Autodesk Inventor part; units mm, degrees
ref_plane "YZ Plane" through (0, 0, 0) normal (1, 0, 0) x (0, 1, 0)
ref_plane "XZ Plane" through (0, 0, 0) normal (0, 1, 0) x (-1, 0, 0)
ref_plane "XY Plane" through (0, 0, 0) normal (0, 0, 1) x (1, 0, 0)
sketch "Sketch1" plane through (0, 0, 0) normal (1, 0, 0) x (0, 1, 0)
  circle A0 centre (0, 0) radius 4.953
  dimension "d0" = 9.906
extrude "Extrusion1" add sketch "Sketch1" along normal blind 0.635
sketch "Sketch2" plane through (0.635, 0, 0) normal (1, 0, 0) x (0, 0, -1)
  circle A0 centre (0, 0) radius 4.953
  circle A1 centre (0, 0) radius 3.4925
  dimension "d3" = 6.985
extrude "Extrusion2" cut sketch "Sketch2" against normal blind 0.381 contours A1
sketch "Sketch3" plane through (0.254, 0, 0) normal (1, 0, 0) x (0, 0, -1)
  circle A0 centre (0, 0) radius 3.4925
hole "Hole1" at (0.254, 0, 0) direction (-1, 0, 0) diameter 4.9022 end through all
properties part number "Washer"
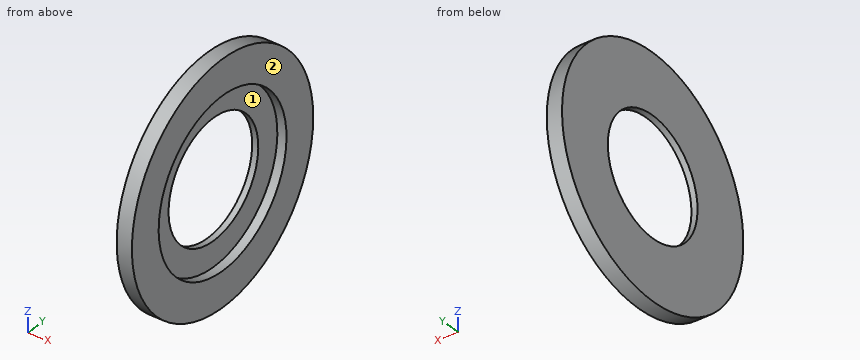
Verification items for the finished model (mm, model axes). Face numbers are marked on the shaded views. A direction names the side the tool comes from. Give positions to 0.01 mm unless a question says otherwise; leave off trailing zeros. Order: outer loops, then holes, each group sorted by start corner. A loop starts at its lowest first (then second) coordinate and runs counter-clockwise, first axis right, second up. Notation, with made-up numbers: (55.25, 63.5) -> (60.25, 63.5) arc R14 ccw to (60.25, 67.5) -> close; hole circle Ø3 at (18, 59). An arc over 180 degrees is marked (long way). Answer as CSV lines item,"result".
Q1. Sectioned sample at C-C on x = 0.45. Record the cut outline in (y, z) (1 decimal).
Solutions:
outline,"circle Ø9.9 at (0, 0); hole circle Ø7 at (0, 0)"
Q2. Depth check by flat-ended pin: pin 1 (2 mm diameter, centred on y = 0, z = 1.5, fed in from +X). Enter the tip coordinate at first touch or a pass-through.
Solutions:
pin 1,"stops at x = 0.25"
Q3. Sectioned sample at D-D on y = -3. Record the cut outline in (x, z) (3 decimals).
Solutions:
outline,"(0, -3.941) -> (0.635, -3.941) -> (0.635, -1.788) -> (0.254, -1.788) -> (0.254, 1.788) -> (0.635, 1.788) -> (0.635, 3.941) -> (0, 3.941) -> close"
Q4. Access from +Z, -Z, +X, -X, +Y, -Y to the whole of each face (thin tool, end or side, straight path). Record for the marked faces 1 and 2.
Solutions:
face 1,"+X"
face 2,"+Z, -Z, +X, +Y, -Y"
Q5. Scan lines: probe 1 along X at (y, z) = (2, 2.25); probe 2 along Y at (x, z) = (0.35, -2.5); probe 3 along Z at (x, y) = (0.35, 1). Record each from-to range of solid material in increasing order.
Solutions:
probe 1,"x = 0 to 0.25"
probe 2,"y = -4.28 to -2.44, 2.44 to 4.28"
probe 3,"z = -4.85 to -3.35, 3.35 to 4.85"
